The figure shows three views and two pictorial views of one solid part (mm, origin at its lowest corner). Answer the questions. Round coordinates to 2 decimals unless told otherwise and drop trailing zeros. Use a Markdown table: item, result. Add a question column.
Q1. Given pin 1 Ø5 at (x, z) = (5, 7.5) entering from +Y; pin 2 Ø1.3 at (y, z) = (23.5, 15) entering from +X; pin 3 Ø4 at (x, z) = (17.5, 16) entering from -Y, each flat-ended and moving along its own axis, determine where each tip first touches the part or whether it passes through.
Q2. Consider line 1 (Z direction, x = 23, y = 2) (1 decimal); line 2 (X direction, y = 14.5, z = 22.5) (1 decimal); line 3 (Y direction, x = 13, z = 16). Determine where each line is inside the solid, lowest interval first.
Q3. For a pull along Y with two mould halves and no side action, classify the marked faces 1, 2 and 3 as released by +Y, released by -Y, zero draft, split by the parting line, or undercut.
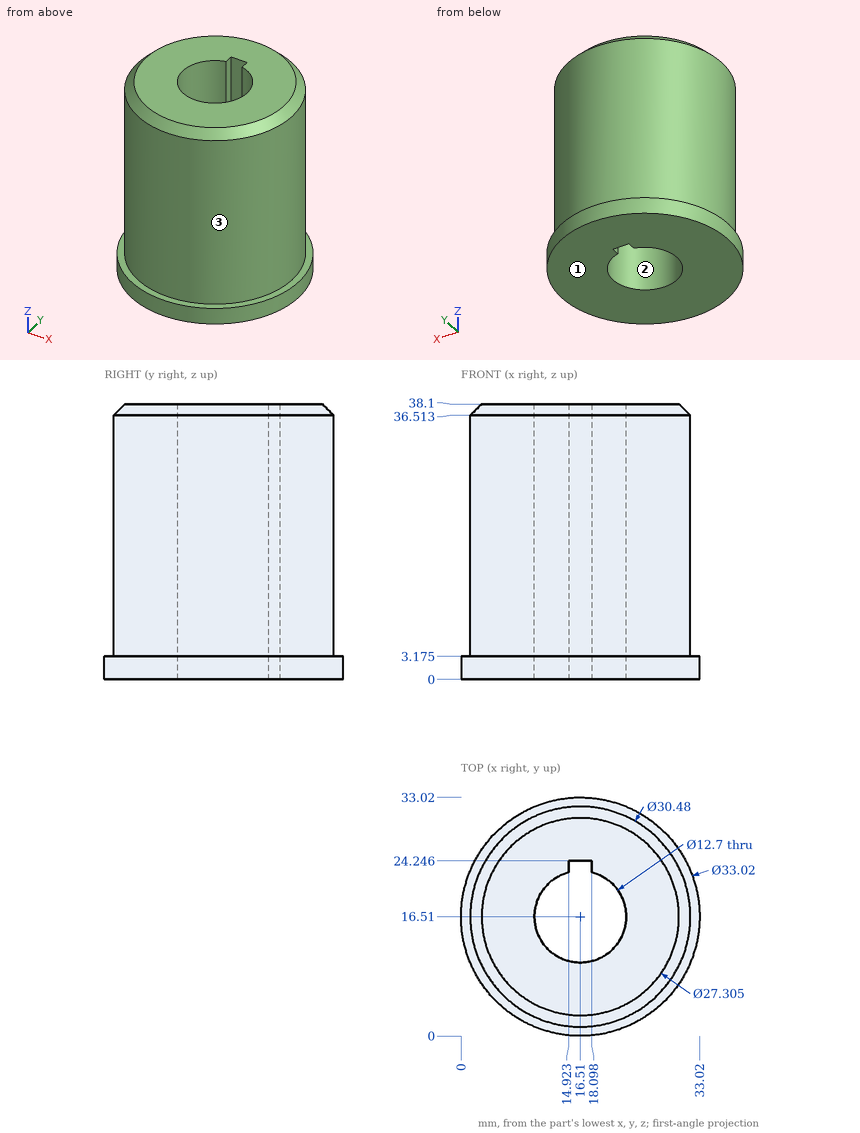
Checked values:
| question | item | result |
|---|---|---|
| 1 | pin 1 | stops at y = 28.8 |
| 1 | pin 2 | stops at x = 30.37 |
| 1 | pin 3 | stops at y = 1.27 |
| 2 | line 1 | z = 0 to 3.2 |
| 2 | line 2 | x = 1.4 to 10.5, 22.5 to 31.6 |
| 2 | line 3 | y = 1.68 to 11.22, 21.8 to 31.34 |
| 3 | face 1 | zero draft |
| 3 | face 2 | undercut |
| 3 | face 3 | split by the parting line |
